Work out the finished part from the listing and answer in its coordinate system (mm). A direction names the side the tool comes from. Coordinates: 2 decimals unless noted, no trailing zeros. Order: outer loops, then holes, each group sorted by start corner. A loop starts at its lowest first (then second) coordinate and runs counter-clockwise, first axis right, second up.
```python
from build123d import *

# Parameters (mm, degrees)
SKETCH_R        = 2.25
PAD_DEPTH       = 3
SKETCH001_W     = 4
SKETCH001_H     = 15
PAD001_DEPTH    = 11
SKETCH002_W     = 5
SKETCH002_H     = 2
POCKET_DEPTH    = 29.501
FILLET_R        = 3
FILLET001_R     = 2
CHAMFER_SIZE    = 0.75
CHAMFER001_SIZE = 2


with BuildPart() as chamfer001:
    # Sketch → Pad (new body)
    with BuildSketch(Plane.XY):
        Polygon((0, 42.65), (-25.5, 42.65), (-29.5, 38.65), (-29.5, 31.65), (-25.5, 27.65), (-14.5, 27.65), (-14.5, 0), (0, 0), align=None)
        with Locations((-23, 35.15)):
            Circle(SKETCH_R, mode=Mode.SUBTRACT)
    extrude(amount=PAD_DEPTH)

    # Sketch001 → Pad001 (new body)
    with BuildSketch(Plane.XY.offset(3)):
        with Locations((-2, 25.5)):
            Rectangle(SKETCH001_W, SKETCH001_H)
    extrude(amount=PAD001_DEPTH)

    # Sketch002 → Pocket (cut, through all)
    with BuildSketch(Plane.YZ):
        with Locations((25.5, 9.8)):
            Rectangle(SKETCH002_W, SKETCH002_H)
    extrude(amount=-POCKET_DEPTH, mode=Mode.SUBTRACT)

    # Fillet
    fillet_edges = [chamfer001.edges().sort_by_distance(p)[0] for p in [
        (-2, 18, 14),
        (-2, 33, 14),
        (-14.5, 0, 1.5),
    ]]
    fillet(fillet_edges, radius=FILLET_R)

    # Fillet001
    fillet001_edges = [chamfer001.edges().sort_by_distance(p)[0] for p in [
        (-4, 25.5, 10.8),
    ]]
    fillet(fillet001_edges, radius=FILLET001_R)

    # Chamfer
    chamfer_edges = [chamfer001.edges().sort_by_distance(p)[0] for p in [
        (0, 21.325, 0),
        (-5.75, 0, 0),
        (-13.62132, 0.87868, 0),
        (-14.5, 15.325, 0),
        (-20, 27.65, 0),
        (-27.5, 29.65, 0),
        (-25.25, 35.15, 0),
    ]]
    chamfer(chamfer_edges, length=CHAMFER_SIZE)

    # Chamfer001
    chamfer001_edges = [chamfer001.edges().sort_by_distance(p)[0] for p in [
        (-2, 18, 3),
        (-4, 25.5, 3),
        (-2, 33, 3),
    ]]
    chamfer(chamfer001_edges, length=CHAMFER001_SIZE)


with BuildPart() as part_mirroring:
    # Part__Mirroring: instance of Chamfer001
    add(chamfer001.part.mirror(Plane(origin=(0, 0, 0), x_dir=(0, -1, 0), z_dir=(1, 0, 0))))


solid = part_mirroring.part
```
1. Flat-ended cylindrical pins translate along their axes: pin 1 (15 mm diameter, centred on x = 15, y = 28.5, fed in from +Z); pin 2 (2 mm diameter, centred on x = 2.5, z = 10.5, fed in from +Y); pin 3 (1.8 mm diameter, centred on y = 14.5, z = 1.5, fed in from +X); pin 4 (1.6 mm diameter, centred on x = 0.5, y = 26.5, fed in from -Z). Find the tip coordinate at first contact, or state that the pin passes through.
2. For faces 4 (the flat face through (2, 33, 8)), 5 (the flat face through (4, 25, 8)), 6 (the flat face through (14.5, 15, 2)), determine the directions among +Z, -Z, +X, -X, +Y, -Y from which every point of the face is accessible in a straight line to the end or side of a thin tool.
3. The part is cut by section B-B (x = 23). Determine the outline of the cut face in (y, z).
4. Consider probe 1 along Y at (x, z) = (23, 1.5); probe 2 along Y at (x, z) = (3.5, 11); probe 3 along X at (y, z) = (29, 8.75). Determine where each line is inside the solid, lowest interval first.
5. The part is cut by section D-D (y = 13). Determine the outline of the cut face in (x, z).
6. The mould has two halves that part along Y. Classify faces 1 (the flat face through (2, 25, 8.8)), 2 (the flat face through (2, 17, 4)), 3 (the flat face through (29.5, 35, 1)): released by +Y, released by -Y, zero draft, split by the parting line, or undercut.
7. The part is cut by section A-A (y = 24). Determine the outline of the cut face in (x, z), plus the area to 3 significant figures.
8. The part is cut by section C-C (x = 3). Determine the outline of the cut face in (y, z).
Worked out:
1. pin 1: stops at z = 3
1. pin 2: stops at y = 33
1. pin 3: stops at x = 14.5
1. pin 4: stops at z = 0
2. face 4: +Z, +X, -X, +Y
2. face 5: +Z, +X, +Y, -Y
2. face 6: +Z, -Z, +X, -Y
3. outline: (27.65, 0.75) - (28.4, 0) - (32.15, 0) - (32.9, 0.75) - (32.9, 3) - (27.65, 3) - close; (37.4, 0.75) - (38.15, 0) - (42.65, 0) - (42.65, 3) - (37.4, 3) - close
4. probe 1: y = 27.65 to 32.9, 37.4 to 42.65
4. probe 2: y = 18 to 23, 28 to 33
4. probe 3: x = 0 to 4
5. outline: (0, 0.75) - (0.75, 0) - (13.75, 0) - (14.5, 0.75) - (14.5, 3) - (0, 3) - close
6. face 1: undercut
6. face 2: released by -Y
6. face 3: zero draft
7. outline: (0, 0.75) - (0.75, 0) - (13.75, 0) - (14.5, 0.75) - (14.5, 3) - (6, 3) - (4, 5) - (4, 8.8) - (0, 8.8) - close; (0, 10.8) - (2, 10.8) arc R2 ccw to (4, 12.8) - (4, 14) - (0, 14) - close
7. area: 80.1 mm2
8. outline: (0, 0.75) - (0.75, 0) - (42.65, 0) - (42.65, 3) - (35, 3) - (33, 5) - (33, 11) arc R3 ccw to (30, 14) - (21, 14) arc R3 ccw to (18, 11) - (18, 5) - (16, 3) - (0, 3) - close; hole (23, 8.8) - (28, 8.8) - (28, 11.07) - (23, 11.07) - close
